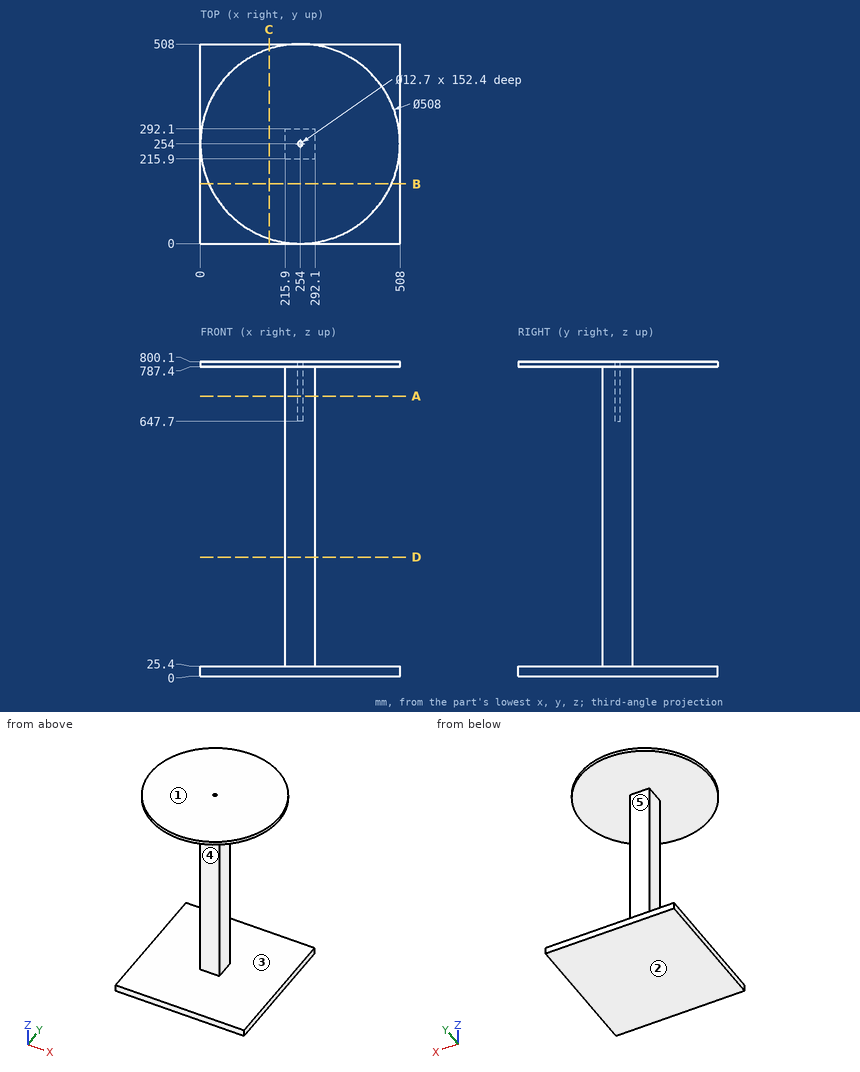
Verification items for this drawing (mm, ordinates from the low corner). A direction names the side the tool comes from. Give positions to 0.01 mm unless a question says otherwise; leave off trailing zeros. Loops run counter-clockwise (first coordinate to the right, second up) from the corner with the lowest first, then second, coordinate; pieces in that order, holes last. Notation, with made-up numbers: M 78,-6 L 83,-6 A31 ccw 83,25 Z; hole C 64.5,28.25 d8. An arc over 180 degrees is marked long. Answer in a Markdown table with one row per item.
1) Mould release check, pull along Z, two halves, no side actions. Record for the marked faces 1, 2 and 3: released by +Z, released by -Z, zero draft, split by the parting line, or undercut.
Solutions:
| item | result |
|---|---|
| face 1 | released by +Z |
| face 2 | released by -Z |
| face 3 | undercut |
2) Thickness scan on line 1 (Z direction, x = 280.5, y = 138.5); line 2 (Y direction, x = 254, z = 716); line 3 (Z direction, x = 79, y = 467). Record the ranges inside material, lowest first.
Solutions:
| item | result |
|---|---|
| line 1 | z = 0 to 25.4, 787.4 to 800.1 |
| line 2 | y = 215.9 to 247.65, 260.35 to 292.1 |
| line 3 | z = 0 to 25.4 |
3) Cross-section at D-D (z = 302.5). Enter the section's corners in (x, y).
Solutions:
| item | result |
|---|---|
| outline | M 215.9,215.9 L 292.1,215.9 L 292.1,292.1 L 215.9,292.1 Z |
4) Tool access check on the marked faces 4 and 5. Record the directions out of +Z, -Z, +X, -X, +Y, -Y that give a thin tool (end or side, any length) a straight path to the whole face; none if there is none.
Solutions:
| item | result |
|---|---|
| face 4 | +X, -X, -Y |
| face 5 | +X, -X, +Y |
5) Cross-section at A-A (z = 712). Enter the section's corners in (x, y).
Solutions:
| item | result |
|---|---|
| outline | M 215.9,215.9 L 292.1,215.9 L 292.1,292.1 L 215.9,292.1 Z; hole C 254,254 d12.7 |
6) Cross-section at B-B (y = 152). Enter the section's corners in (x, z).
Solutions:
| item | result |
|---|---|
| outline | M 0,0 L 508,0 L 508,25.4 L 0,25.4 Z; M 21.38,787.4 L 486.62,787.4 L 486.62,800.1 L 21.38,800.1 Z |
7) Cross-section at C-C (x = 175). Enter the section's corners in (y, z), plus the area to 3 significant figures.
Solutions:
| item | result |
|---|---|
| outline | M 0,0 L 508,0 L 508,25.4 L 0,25.4 Z; M 12.6,787.4 L 495.4,787.4 L 495.4,800.1 L 12.6,800.1 Z |
| area | 19,000 mm^2 |
8) Depth check by flat-ended pin: pin 1 (6 mm diameter, centred on x = 279, z = 282, fed in from -Y); pin 2 (8 mm diameter, centred on x = 291, z = 523.5, fed in from +Y); pin 3 (11.5 mm diameter, centred on x = 254, y = 254, fed in from +Z). Enter the tip coordinate at first touch or a pass-through.
Solutions:
| item | result |
|---|---|
| pin 1 | stops at y = 215.9 |
| pin 2 | stops at y = 292.1 |
| pin 3 | stops at z = 647.7 |
